Drawing for the job (mm, zero at the part's lowest x, y, z). A direction names the side the tool comes from. Coordinates: 2 decimals unless noted, no trailing zeros. Write each loop counter-clockwise with the first axis right and the second up, starting at its lowest first coordinate (ties: lowest second). Pieces come first, ordered by that corner, then holes. Notation, with made-up numbers: (42.25, -39.5) - (46.25, -39.5) arc R17 cw to (46.25, -34.5) - close; hole circle Ø11 at (-0.75, 67.5). An arc over 180 degrees is marked (long way). Write each question's results on one line, items separated by ' | '.
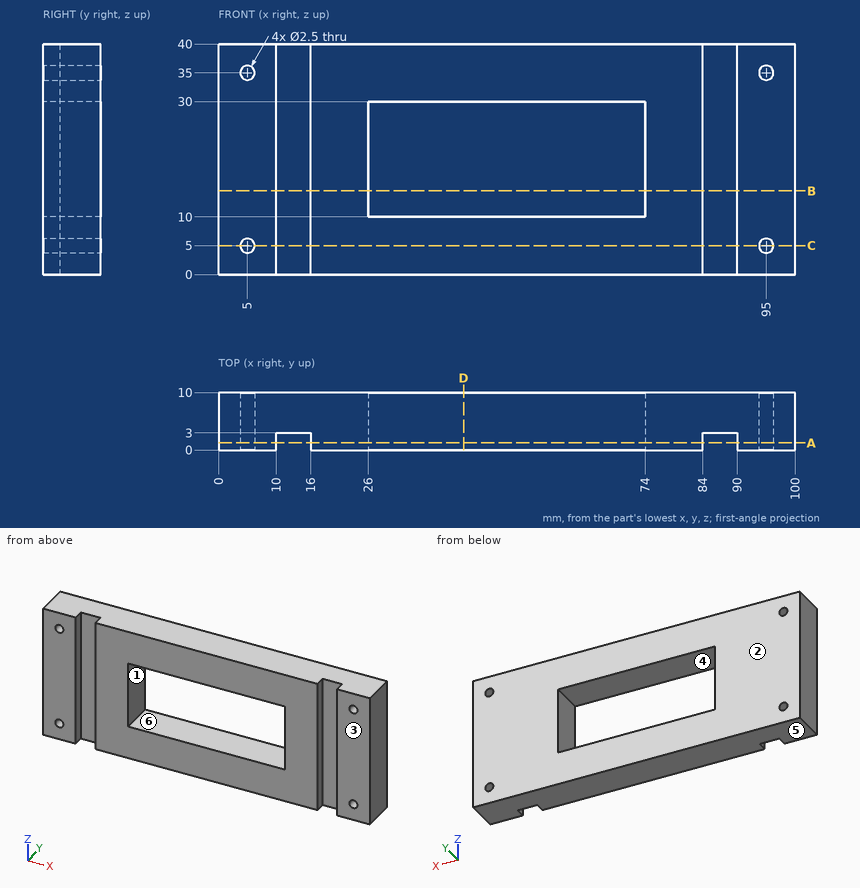
(1) Saw through at D-D on x = 42.5. Write the cut outline in (y, z), then the cut area to 3 significant figures.
Return value:
outline: (0, 0) - (10, 0) - (10, 10) - (0, 10) - close; (0, 30) - (10, 30) - (10, 40) - (0, 40) - close | area: 200 mm^2
(2) 3-axis set-ups, long thin cutter, end or side, ignore diameter. For the marked faces 1 and 2: which of +Z, -Z, +X, -X, +Y, -Y reach the whole face in a straight line?
Return value:
face 1: +Y, -Y | face 2: +Z, -Z, +X, -X, +Y
(3) Wall check: line 1 (X direction, y = 1.5, z = 12.5); line 2 (Z direction, x = 95, y = 4); line 3 (X direction, y = 8, z = 5). Give the ranges that are in metal, low to high. Write a range as from..to.
Return value:
line 1: x = 0..10, 16..26, 74..84, 90..100 | line 2: z = 0..3.75, 6.25..33.75, 36.25..40 | line 3: x = 0..3.75, 6.25..93.75, 96.25..100
(4) Saw through at C-C on z = 5. Write the cut outline in (x, y), then the cut area to 3 significant figures.
Return value:
outline: (0, 0) - (3.75, 0) - (3.75, 10) - (0, 10) - close; (6.25, 0) - (10, 0) - (10, 3) - (16, 3) - (16, 0) - (84, 0) - (84, 3) - (90, 3) - (90, 0) - (93.75, 0) - (93.75, 10) - (6.25, 10) - close; (96.25, 0) - (100, 0) - (100, 10) - (96.25, 10) - close | area: 914 mm^2
(5) Saw through at A-A on y = 1.25. Write the cut outline in (x, z).
Return value:
outline: (0, 0) - (10, 0) - (10, 40) - (0, 40) - close; (16, 0) - (84, 0) - (84, 40) - (16, 40) - close; (90, 0) - (100, 0) - (100, 40) - (90, 40) - close; hole circle Ø2.5 at (5, 5); hole circle Ø2.5 at (5, 35); hole (26, 10) - (74, 10) - (74, 30) - (26, 30) - close; hole circle Ø2.5 at (95, 5); hole circle Ø2.5 at (95, 35)
(6) Two-plate mould, pull along Z, no slides. Class the marked faces 3, 4, 5 and 6: released by +Z, released by -Z, zero draft, split by the parting line, or undercut.
Return value:
face 3: zero draft | face 4: undercut | face 5: released by -Z | face 6: undercut
(7) Saw through at B-B on z = 14.5. Write the cut outline in (x, y), then the cut area to 3 significant figures.
Return value:
outline: (0, 0) - (10, 0) - (10, 3) - (16, 3) - (16, 0) - (26, 0) - (26, 10) - (0, 10) - close; (74, 0) - (84, 0) - (84, 3) - (90, 3) - (90, 0) - (100, 0) - (100, 10) - (74, 10) - close | area: 484 mm^2
(8) Flat gauge pin, fed straight in: P1, Ø3, axis at x = 86.5, z = 14, coming from the -Y side. Where does the tip first touch, or does it go through?
Return value:
P1: stops at y = 3
